Verification items for the finished model (mm, model axes). Give positions to 0.01 mm unless a question says otherwise; leave off trailing zeros. Order: outer loops, then holes, each group sorted by start corner. A loop starts at its lowest first (then second) coordinate and runs counter-clockwise, first axis right, second up. Notation, with made-up numbers: (-17.5, -34.5) - (25.5, -34.5) arc R9 cw to (25.5, -22.5) - close; hole circle Ø11 at (-33, -28.5). An arc over 180 degrees is marked (long way). Answer as a JSON object with one key per item and string values. Group by question number.
(1) Section check C-C (z = 31). Count the separate pieces of the cut face and the enclosed holes in it, then the cut area to 3 significant figures.
(2) Thickness scan on line 1 (Y direction, x = 98.5, z = 16); line 2 (Z direction, x = 6, y = 50). Record the ranges inside material, lowest first.
(3) Section check A-A (x = 123). Record the boundary of the cut face in (y, z).
(4) Depth check by flat-ended pin: pin 1 Ø10 at (y, z) = (112, 18) entering from -X; pin 2 Ø1.9 at (x, y) = (52, 53) entering from +Z; pin 3 Ø1.9 at (x, y) = (130, 53.5) entering from +Z. Enter the tip coordinate at first touch or a pass-through.
```python
from build123d import *

# Parameters (mm, degrees)
F0_W      = 152.4
F0_H      = 152.4
F1_DEPTH  = 35.9833333333
F2_W      = 42.3333333333
F2_H      = 29.6333333333
F3_DEPTH  = 396.24
F4_W      = 42.3333333333
F4_H      = 29.6333333333
F5_DEPTH  = 206.248
F6_W      = 42.3333333333
F6_H      = 42.3333333333
F7_DEPTH  = 25.4
F8_R      = 2.413
F9_DEPTH  = 5.08
F10_R     = 2.54
F11_DEPTH = 3.81
F12_R     = 1.27


with BuildPart() as f1:
    # F0 (on Top) → F1 (new body)
    with BuildSketch(Plane.XY):
        with Locations((76.2, 76.2)):
            Rectangle(F0_W, F0_H)
    extrude(amount=F1_DEPTH)

    # F2 (on face) → F3 (cut)
    with BuildSketch(Plane.XZ):
        with Locations((27.5166666667, 21.1666666667)):
            Rectangle(F2_W, F2_H)
        with Locations((76.2, 21.1666666667)):
            Rectangle(F2_W, F2_H)
        with Locations((124.8833333333, 21.1666666667)):
            Rectangle(F2_W, F2_H)
    extrude(amount=-F3_DEPTH, mode=Mode.SUBTRACT)

    # F4 (on face) → F5 (cut)
    with BuildSketch(Plane.YZ.offset(152.4)):
        with Locations((27.5166666667, 21.1666666667)):
            Rectangle(F4_W, F4_H)
        with Locations((76.2, 21.1666666667)):
            Rectangle(F4_W, F4_H)
        with Locations((124.8833333333, 21.1666666667)):
            Rectangle(F4_W, F4_H)
    extrude(amount=-F5_DEPTH, mode=Mode.SUBTRACT)

    # F6 (on face) → F7 (cut)
    with BuildSketch(Plane.XY.offset(6.35)):
        with Locations((27.5166666667, 124.8833333333)):
            Rectangle(F6_W, F6_H)
        with Locations((76.2, 124.8833333333)):
            Rectangle(F6_W, F6_H)
        with Locations((124.8833333333, 124.8833333333)):
            Rectangle(F6_W, F6_H)
        with Locations((27.5166666667, 76.2)):
            Rectangle(F6_W, F6_H)
        with Locations((76.2, 76.2)):
            Rectangle(F6_W, F6_H)
        with Locations((124.8833333333, 76.2)):
            Rectangle(F6_W, F6_H)
        with Locations((27.5166666667, 27.5166666667)):
            Rectangle(F6_W, F6_H)
        with Locations((76.2, 27.5166666667)):
            Rectangle(F6_W, F6_H)
        with Locations((124.8833333333, 27.5166666667)):
            Rectangle(F6_W, F6_H)
    extrude(amount=-F7_DEPTH, mode=Mode.SUBTRACT)

    # F8 (on face) → F9 (join)
    with BuildSketch(Plane.XY.offset(35.9833333333)):
        with Locations((149.225, 3.175)):
            Circle(F8_R)
    extrude(amount=F9_DEPTH)

    # F10 (on face) → F11 (join)
    with BuildSketch(Plane.XY.offset(41.0633333333)):
        with Locations((149.225, 3.175)):
            Circle(F10_R)
    extrude(amount=F11_DEPTH)

    # F12
    f12_edges = [f1.edges().sort_by_distance(p)[0] for p in [
        (146.685, 3.175, 44.873333),
    ]]
    fillet(f12_edges, radius=F12_R)


solid = f1.part
```
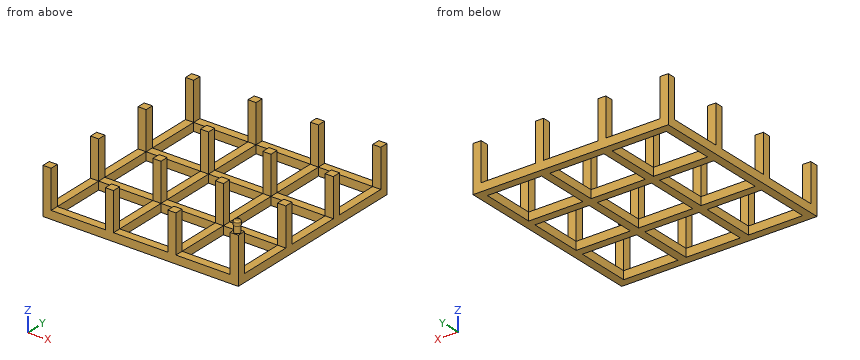
Solutions:
{
 "1": {"separate pieces": "16", "enclosed holes": "0", "area": "645 mm2"},
 "2": {"line 1": "y = 0 to 6.35, 48.68 to 55.03, 97.37 to 103.72, 146.05 to 152.4", "line 2": "z = 0 to 35.98"},
 "3": {"outline": "(0, 0) - (6.35, 0) - (6.35, 6.35) - (0, 6.35) - close; (48.68, 0) - (55.03, 0) - (55.03, 6.35) - (48.68, 6.35) - close; (97.37, 0) - (103.72, 0) - (103.72, 6.35) - (97.37, 6.35) - close; (146.05, 0) - (152.4, 0) - (152.4, 6.35) - (146.05, 6.35) - close"},
 "4": {"pin 1": "passes through", "pin 2": "stops at z = 35.98", "pin 3": "stops at z = 6.35"}
}
